Can you work these out from the model? Positions are in its coordinate system, mm. A direction names the side the tool comes from. Round coordinates to 2 decimals unless told otherwise and drop trailing zeros. Loops run counter-clockwise (first coordinate to the right, second up) from the corner with the lowest first, then second, coordinate; pieces in that order, holes last.
(1) Will these pins go through, and if not, where does the flat tip stop? pin 1 Ø1 at (x, z) = (-16.5, 59) entering from +Y; pin 2 Ø1.5 at (x, z) = (-17, -55.5) entering from -Y; pin 3 Ø2 at (y, z) = (1.5, 60.5) entering from -X.
(2) If I drill on line 1 along X through (y, z) = (4.5, 0); line 2 along X through (y, z) = (-69, -17); line 3 along Y through (x, z) = (-34.5, -14.5), over which ranges is the centre line in solid material (lowest first)?
(3) Thinking about a two-plate mould opening in Z: for faces 3 (the face through (77, 4, 0)), 4 (the face through (-34.277, -49.3, -18.021)), 5 (the face through (-4.88, 3.94, -1.08)), 6 (the face through (30, -100, -18)), which applies, released by +Z, released by -Z, zero draft, split by the parting line, or undercut?
(4) I want a section at A-A on z = -17.5. Write out the boundary of the cut face in (x, y), plus the area to 3 significant figures.
(5) Which directions (+Z, -Z, +X, -X, +Y, -Y) give clear straight access to the entire face, cutting with the end or side of a thin tool? Please do faces 1 (the face through (0.66, 11.944, -14.985)), 2 (the face through (-78.1, 3.94, -17.34)).
(6) I want a section at B-B on y = -86.5. Write out the boundary of the cut face in (x, z), plus the area to 3 significant figures.
(7) I want a section at C-C on z = -59. Write out the boundary of the cut face in (x, y), plus the area to 3 significant figures.
from build123d import *

# Parameters (mm, degrees)
CROQUIS1_R              = 80
CROQUIS1_R_2            = 5
SALIENTE_EXTRUIR1_DEPTH = 8
CROQUIS2_R              = 2
CORTAR_EXTRUIR1_DEPTH   = 10
CROQUIS3_R              = 35
CROQUIS3_R_2            = 30
CROQUIS3_R_3            = 15
CROQUIS3_R_4            = 12.15
SALIENTE_EXTRUIR2_DEPTH = 8
CROQUIS4_R              = 35
CROQUIS4_R_2            = 30
SALIENTE_EXTRUIR3_DEPTH = 10
CROQUIS5_R              = 4
SALIENTE_EXTRUIR4_DEPTH = 100


with BuildPart() as part:
    # Croquis1 → Saliente-Extruir1 (new body)
    with BuildSketch(Plane(origin=(0, 0, 0), x_dir=(1, 0, 0), z_dir=(0, 1, 0))):
        with Locations(Location((0, 0, 0), (0, 0, 270))):
            Circle(CROQUIS1_R)
        with Locations(Location((0, 0, 0), (0, 0, 270))):
            Circle(CROQUIS1_R_2, mode=Mode.SUBTRACT)
    extrude(amount=SALIENTE_EXTRUIR1_DEPTH)

    # Croquis2 → Cortar-Extruir1 (cut)
    with BuildSketch(Plane(origin=(0, 8, 0), x_dir=(1, 0, 0), z_dir=(0, 1, 0))):
        with Locations(Location((0, 75, 0), (0, 0, 270))):
            Circle(CROQUIS2_R)
        with Locations(Location((53.033008589, 53.033008589, 0), (0, 0, 270))):
            Circle(CROQUIS2_R)
        with Locations(Location((75, 0, 0), (0, 0, 270))):
            Circle(CROQUIS2_R)
        with Locations(Location((53.033008589, -53.033008589, 0), (0, 0, 270))):
            Circle(CROQUIS2_R)
        with Locations(Location((0, -75, 0), (0, 0, 270))):
            Circle(CROQUIS2_R)
        with Locations(Location((-53.033008589, -53.033008589, 0), (0, 0, 270))):
            Circle(CROQUIS2_R)
        with Locations(Location((-75, 0, 0), (0, 0, 270))):
            Circle(CROQUIS2_R)
        with Locations(Location((-53.033008589, 53.033008589, 0), (0, 0, 270))):
            Circle(CROQUIS2_R)
    extrude(amount=-CORTAR_EXTRUIR1_DEPTH, mode=Mode.SUBTRACT)

    # Croquis3 → Saliente-Extruir2 (add)
    # profile 1 of 2: a face of its own
    with BuildSketch(Plane(origin=(0, 8, 0), x_dir=(1, 0, 0), z_dir=(0, 1, 0))):
        with Locations(Location((0, 0, 0), (0, 0, 270))):
            Circle(CROQUIS3_R)
        with Locations(Location((0, 0, 0), (0, 0, 270))):
            Circle(CROQUIS3_R_2, mode=Mode.SUBTRACT)
    # profile 2 of 2: a face of its own
    with BuildSketch(Plane(origin=(0, 8, 0), x_dir=(1, 0, 0), z_dir=(0, 1, 0))):
        with Locations(Location((0, 0, 0), (0, 0, 270))):
            Circle(CROQUIS3_R_3)
        with Locations(Location((0, 0, 0), (0, 0, 270))):
            Circle(CROQUIS3_R_4, mode=Mode.SUBTRACT)
    extrude(amount=SALIENTE_EXTRUIR2_DEPTH)

    # Croquis4 → Saliente-Extruir3 (add)
    with BuildSketch(Plane(origin=(0, 16, 0), x_dir=(1, 0, 0), z_dir=(0, 1, 0))):
        with Locations(Location((0, 0, 0), (0, 0, 270))):
            Circle(CROQUIS4_R)
        with Locations(Location((0, 0, 0), (0, 0, 270))):
            Circle(CROQUIS4_R_2, mode=Mode.SUBTRACT)
    extrude(amount=SALIENTE_EXTRUIR3_DEPTH)

    # Croquis5 → Saliente-Extruir4 (add)
    with BuildSketch(Plane.XZ):
        with Locations(Location((0, 35, 0), (0, 0, 90))):
            Circle(CROQUIS5_R)
        with Locations(Location((30.310889132, -17.5, 0), (0, 0, 90))):
            Circle(CROQUIS5_R)
        with Locations(Location((-30.310889132, -17.5, 0), (0, 0, 90))):
            Circle(CROQUIS5_R)
    extrude(amount=SALIENTE_EXTRUIR4_DEPTH)


solid = part.part
Filled sheet:
1. pin 1: stops at y = 8
1. pin 2: stops at y = 0
1. pin 3: stops at x = -53.48
2. line 1: x = -80 to -77, -73 to -5, 5 to 73, 77 to 80
2. line 2: x = -34.28 to -26.34, 26.34 to 34.28
2. line 3: y = 0 to 8
3. face 3: undercut
3. face 4: split by the parting line
3. face 5: undercut
3. face 6: zero draft
4. outline: (-78.06, 0) - (-34.31, 0) - (-34.31, -100) - (-26.31, -100) - (-26.31, 0) - (26.31, 0) - (26.31, -100) - (34.31, -100) - (34.31, 0) - (78.06, 0) - (78.06, 8) - (30.31, 8) - (30.31, 26) - (24.37, 26) - (24.37, 8) - (-24.37, 8) - (-24.37, 26) - (-30.31, 26) - (-30.31, 8) - (-78.06, 8) - close
4. area: 3,060 mm2
5. face 1: +Y
5. face 2: +Y, -Y
6. outline: circle Ø8 at (-30.31, -17.5); circle Ø8 at (0, 35); circle Ø8 at (30.31, -17.5)
6. area: 151 mm2
7. outline: (-54.03, 0) - (54.03, 0) - (54.03, 8) - (-54.03, 8) - close
7. area: 864 mm2
